```python
from build123d import *

# Parameters (mm, degrees)
CYLINDER020_R     = 5
CYLINDER020_DEPTH = 5
CYLINDER019_R     = 5
CYLINDER019_DEPTH = 5
BOX005_W          = 15
BOX005_H          = 2
BOX005_DEPTH      = 20
FILLET002_R       = 2
BOX002_W          = 10
BOX002_H          = 2
BOX002_DEPTH      = 20
BOX_W             = 80
BOX_H             = 39
BOX_DEPTH         = 25
CYLINDER002_R     = 31.75
CYLINDER002_DEPTH = 25
BOX001_W          = 7.7
BOX001_H          = 7.7
BOX001_DEPTH      = 10
BOX007_W          = 72
BOX007_H          = 42
BOX007_DEPTH      = 2
CYLINDER_R        = 31.75
CYLINDER_DEPTH    = 18
CYLINDER001_R     = 34.5
CYLINDER001_DEPTH = 20
FILLET001_R       = 2
BOX006_W          = 15
BOX006_H          = 2
BOX006_DEPTH      = 20
FILLET003_R       = 2


with BuildPart() as cylinder020:
    # Cylinder020 → Cylinder020 (new body)
    with BuildSketch(Plane(origin=(-39.01, -14.6034, 15), x_dir=(1, 0, 0), z_dir=(0, 0, 1))):
        Circle(CYLINDER020_R)
    extrude(amount=CYLINDER020_DEPTH)


with BuildPart() as fusion013:
    # Cylinder019 → Cylinder019 (new body)
    with BuildSketch(Plane(origin=(38.99, -14.6034, 15), x_dir=(1, 0, 0), z_dir=(0, 0, 1))):
        Circle(CYLINDER019_R)
    extrude(amount=CYLINDER019_DEPTH)

    # Fusion013: union Cylinder020
    add(cylinder020.part)


with BuildPart() as fillet002:
    # Box005 → Box005 (new body)
    with BuildSketch(Plane(origin=(31.79, 6.35995, 0), x_dir=(1, 0, 0), z_dir=(0, 0, 1))):
        with Locations((7.5, 1)):
            Rectangle(BOX005_W, BOX005_H)
    extrude(amount=BOX005_DEPTH)

    # Fillet002
    fillet002_edges = [fillet002.edges().sort_by_distance(p)[0] for p in [
        (46.79, 7.35995, 20),
        (46.79, 7.35995, 0),
    ]]
    fillet(fillet002_edges, radius=FILLET002_R)


with BuildPart() as kostka002:
    # Box002 → Box002 (new body)
    with BuildSketch(Plane(origin=(31.22162, 4.362905, 0), x_dir=(1, 0, 0), z_dir=(0, 0, 1))):
        with Locations((5, 1)):
            Rectangle(BOX002_W, BOX002_H)
    extrude(amount=BOX002_DEPTH)


with BuildPart() as kostka:
    # Box → Box (new body)
    with BuildSketch(Plane(origin=(-38, -32.5, 0), x_dir=(1, 0, 0), z_dir=(0, 0, 1))):
        with Locations((40, 19.5)):
            Rectangle(BOX_W, BOX_H)
    extrude(amount=BOX_DEPTH)


with BuildPart() as cut001:
    # Cylinder002 → Cylinder002 (new body)
    with BuildSketch(Plane.XY):
        Circle(CYLINDER002_R)
    extrude(amount=CYLINDER002_DEPTH)

    # Cut001: cut Kostka
    add(kostka.part, mode=Mode.SUBTRACT)


with BuildPart() as kostka001:
    # Box001 → Box001 (new body)
    with BuildSketch(Plane(origin=(25.1, -7, 10), x_dir=(0, 1, 0), z_dir=(0, 0, 1))):
        with Locations((3.85, 3.85)):
            Rectangle(BOX001_W, BOX001_H)
    extrude(amount=BOX001_DEPTH)


with BuildPart() as kostka007:
    # Box007 → Box007 (new body)
    with BuildSketch(Plane(origin=(-36.01, -35.6034, 18), x_dir=(1, 0, 0), z_dir=(0, 0, 1))):
        with Locations((36, 21)):
            Rectangle(BOX007_W, BOX007_H)
    extrude(amount=BOX007_DEPTH)


with BuildPart() as cylinder:
    # Cylinder → Cylinder (new body)
    with BuildSketch(Plane.XY):
        Circle(CYLINDER_R)
    extrude(amount=CYLINDER_DEPTH)


with BuildPart() as fusion001:
    # Cylinder001 → Cylinder001 (new body)
    with BuildSketch(Plane.XY):
        Circle(CYLINDER001_R)
    extrude(amount=CYLINDER001_DEPTH)

    # Cut: cut Cylinder
    add(cylinder.part, mode=Mode.SUBTRACT)

    # Fusion: union Kostka007
    add(kostka007.part)

    # Cut002: cut Kostka001
    add(kostka001.part, mode=Mode.SUBTRACT)

    # Cut003: cut Cut001
    add(cut001.part, mode=Mode.SUBTRACT)

    # Cut004: cut Kostka002
    add(kostka002.part, mode=Mode.SUBTRACT)

    # Fillet001
    fillet001_edges = [fusion001.edges().sort_by_distance(p)[0] for p in [
        (-36.01, -35.6034, 19),
        (35.99, -35.6034, 19),
    ]]
    fillet(fillet001_edges, radius=FILLET001_R)

    # Fusion001: union Fillet002
    add(fillet002.part)


with BuildPart() as base:
    # Box006 → Box006 (new body)
    with BuildSketch(Plane(origin=(31.7936, 2.359946, 0), x_dir=(1, 0, 0), z_dir=(0, 0, 1))):
        with Locations((7.5, 1)):
            Rectangle(BOX006_W, BOX006_H)
    extrude(amount=BOX006_DEPTH)

    # Fillet003
    fillet003_edges = [base.edges().sort_by_distance(p)[0] for p in [
        (46.7936, 3.359946, 20),
        (46.7936, 3.359946, 0),
    ]]
    fillet(fillet003_edges, radius=FILLET003_R)

    # Fusion002: union Fusion001
    add(fusion001.part)

    # Cut015: cut Fusion013
    add(fusion013.part, mode=Mode.SUBTRACT)


solid = base.part
```
Verification items for the finished model (mm, model axes). A direction names the side the tool comes from. Coordinates: 2 decimals unless noted, no trailing zeros. Order: outer loops, then holes, each group sorted by start corner. A loop starts at its lowest first (then second) coordinate and runs counter-clockwise, first axis right, second up. Notation, with made-up numbers: (10, -14.75) -> (34, -14.75) arc R11 cw to (34, -6.75) -> close; hole circle Ø1 at (33, 45.25). An arc over 180 degrees is marked (long way). Answer as CSV lines item,"result". Start each with the question number.
1) Cross-section at B-B, the plane y = 23. Record the boundary of the cut face in (x, z).
2) Cross-section at A-A, the plane x = 0. Record the boundary of the cut face in (y, z).
3) Set-up check for faces 5 (the face through (-35, 6.397, 19)), 6 (the face through (17.4, -3, 19)), 7 (the face through (33, 4.363, 10)), 8 (the face through (0, -8, 18)): record each of +Z, -Z, +X, -X, +Y, -Y from which the full face is reachable in a straight line by a thin tool's end or side.
4) Gauge pin test, flat ends, axial feed: pin 1 Ø4 at (y, z) = (-19.5, 2.5) entering from -X; pin 2 Ø0.5 at (x, z) = (31.5, 5.5) entering from -Y; pin 3 Ø0.6 at (y, z) = (5, 10.5) entering from +X; pin 4 Ø5 at (x, y) = (4.5, 27) entering from +Z. Record the tip position at first contact, or that the pin passes through.
5) Cross-section at C-C, the plane x = 24. Record the boundary of the cut face in (y, z), then the cut area to 3 significant figures.
6) Release check for a two-part mould opening along Y. For faces 1 (the face through (33.99, -14.54, 18.99)), 2 (the face through (40, 8.36, 10)), 3 (the face through (35.42, -35, 19.01)), 4 (the face through (46.22, 3.37, 0.6)) record: released by +Y, released by -Y, zero draft, split by the parting line, or undercut.
7) Material ranges on L1, parallel to Y at x = 0, z = 6.5; L2, parallel to Y at x = 36, z = 12.25, recorded low to high. Write a range as [from, to].
Conclusion:
1,outline,"(-25.71, 0) -> (-21.89, 0) -> (-21.89, 20) -> (-25.71, 20) -> close; (21.89, 0) -> (25.71, 0) -> (25.71, 20) -> (21.89, 20) -> close"
2,outline,"(-35.6, 18) -> (-34.5, 18) -> (-34.5, 0) -> (-31.75, 0) -> (-31.75, 18) -> (6.5, 18) -> (6.5, 20) -> (-35.6, 20) -> close; (31.75, 0) -> (34.5, 0) -> (34.5, 20) -> (31.75, 20) -> close"
3,face 5,"+Z, -Z, -X, +Y"
3,face 6,"+Z, -Z"
3,face 7,"+Z, -Z, +X"
3,face 8,"-Z"
4,pin 1,"stops at x = -29.73"
4,pin 2,"stops at y = -14.62"
4,pin 3,"stops at x = -31.3"
4,pin 4,"passes through"
5,outline,"(-35.6, 18) -> (-24.78, 18) -> (-24.78, 0) -> (-20.79, 0) -> (-20.79, 18) -> (-7, 18) -> (-7, 20) -> (-35.6, 20) -> close; (0.7, 18) -> (6.5, 18) -> (6.5, 20) -> (0.7, 20) -> close; (20.79, 0) -> (24.78, 0) -> (24.78, 20) -> (20.79, 20) -> close"
5,area,"221 mm²"
6,face 1,"undercut"
6,face 2,"released by +Y"
6,face 3,"released by -Y"
6,face 4,"zero draft"
7,L1,"y = [-34.5, -31.75], [31.75, 34.5]"
7,L2,"y = [2.36, 4.36], [6.36, 8.36]"
